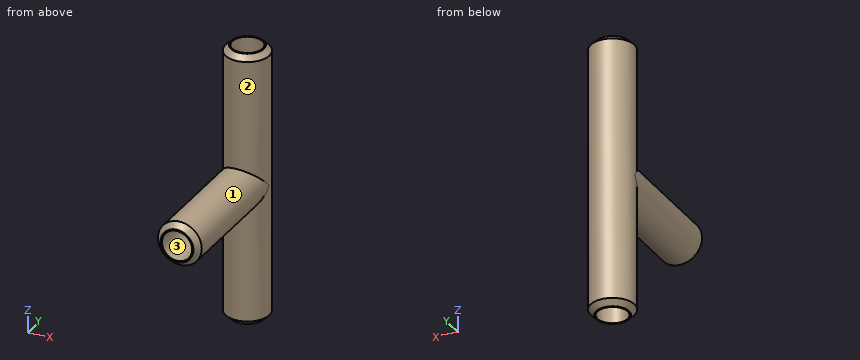
from build123d import *

# Parameters (mm, degrees)
SKETCH_R        = 4
PAD_DEPTH       = 50
SKETCH001_R     = 4
PAD001_DEPTH    = 25
SKETCH002_R     = 2.75
POCKET_DEPTH    = 50.001
SKETCH003_R     = 2.75
POCKET001_DEPTH = 25
CHAMFER_SIZE    = 1


with BuildPart() as part:
    # Sketch → Pad (new body)
    with BuildSketch(Plane.XY):
        Circle(SKETCH_R)
    extrude(amount=PAD_DEPTH)

    # Sketch001 → Pad001 (join)
    with BuildSketch(Plane.XZ):
        with Locations((0, 25)):
            Circle(SKETCH001_R)
    extrude(amount=PAD001_DEPTH)

    # Sketch002 (on Face2 of Pad001) → Pocket (cut, through all)
    with BuildSketch(Plane(origin=(0, 0, 0), x_dir=(1, 0, 0), z_dir=(0, 0, -1))):
        Circle(SKETCH002_R)
    extrude(amount=-POCKET_DEPTH, mode=Mode.SUBTRACT)

    # Sketch003 (on Face6 of Pocket) → Pocket001 (cut)
    with BuildSketch(Plane.XZ.offset(25)):
        with Locations((0, 25)):
            Circle(SKETCH003_R)
    extrude(amount=-POCKET001_DEPTH, mode=Mode.SUBTRACT)

    # Chamfer
    chamfer_edges = [part.edges().sort_by_distance(p)[0] for p in [
        (-4, 0, 0),
        (-4, -25, 25),
        (-4, 0, 50),
    ]]
    chamfer(chamfer_edges, length=CHAMFER_SIZE)


solid = part.part
Source: CAD feature listing. Evaluate the final solid. Frame: model axes, mm. Face numbers are marked on the shaded views. Give positions to 0.01 mm unless a question says otherwise; leave off trailing zeros. Write each loop counter-clockwise with the first axis right and the second up, starting at its lowest first coordinate (ties: lowest second). Pieces come first, ordered by that corner, then holes. Notation, with made-up numbers: M 71,80 L 90,80 A19 cw 90,112 Z; hole C 9.25,43.25 d2. An arc over 180 degrees is marked long. Return JSON: item names as keys, results as strings. Group by question number.
1) Pin query (flat end, axial travel): P1, Ø1, axis at x = -2.5, y = -8.5, coming from the -Z side; P2, Ø3, axis at x = -3, z = 31.5, coming from the +Y side; P3, Ø1.5, axis at x = -2, z = 40.5, coming from the -Y side. Return the tip coordinate at first contact, or that it passes through.
2) Pull-direction query (Z, two-part tool) for the marked faces 1, 2 and 3; classes: pulls with the +Z half, pulls with the -Z half, needs draft (parallel to the pull), parting line crosses it, or undercut.
3) Cut plane C-C, the plane y = -13. Output: boundary loops of the cut face in (x, z).
4) Cut plane A-A, the plane x = 0. Output: boundary loops of the cut face in (y, z).
5) Cut plane B-B, the plane z = 25. Output: boundary loops of the cut face in (x, y), plus the area to 3 significant figures.
6) Cut plane D-D, the plane z = 12. Output: boundary loops of the cut face in (x, y).
7) Material intervals for line 1 along Z through (x, y) = (0, -14.25); line 2 along X through (y, z) = (0, 39.5), sorted ascending. Write a range as [from, to].
Recorded:
{
 "1": {"P1": "stops at z = 21.54", "P2": "stops at y = 3.71", "P3": "stops at y = -3.8"},
 "2": {"face 1": "parting line crosses it", "face 2": "needs draft", "face 3": "undercut"},
 "3": {"outline": "C 0,25 d8; hole C 0,25 d5.5"},
 "4": {"outline": "M -25,22 L -24,21 L -4,21 L -4,1 L -3,0 L -2.75,0 L -2.75,22.25 L -25,22.25 Z; M -25,27.75 L -2.75,27.75 L -2.75,50 L -3,50 L -4,49 L -4,29 L -24,29 L -25,28 Z; M 2.75,0 L 3,0 L 4,1 L 4,49 L 3,50 L 2.75,50 Z"},
 "5": {"outline": "M -4,-24 L -3,-25 L -2.75,-25 L -2.75,0 A2.75 cw 2.75,0 L 2.75,-25 L 3,-25 L 4,-24 L 4,0 A4 ccw -4,0 Z", "area": "74.8 mm²"},
 "6": {"outline": "C 0,0 d8; hole C 0,0 d5.5"},
 "7": {"line 1": "z = [21, 22.25], [27.75, 29]", "line 2": "x = [-4, -2.75], [2.75, 4]"}
}
